Geometry: final body of the model. Coordinates: model frame, mm. A direction names the side the tool comes from. Round coordinates to 2 decimals unless told otherwise and drop trailing zeros. Write each loop counter-clockwise with the first axis right and the second up, starting at its lowest first coordinate (ties: lowest second). Pieces come first, ordered by that corner, then holes.
from build123d import *

# Parameters (mm, degrees)
SKETCH1_R               = 22.5
BOSS_EXTRUDE1_DEPTH     = 50
CUT_EXTRUDE1_REACH      = 130.311
CUT_EXTRUDE1_END_RADIUS = 22.5
SKETCH2_R               = 5


with BuildPart() as part:
    # Sketch1 → Boss-Extrude1 (new body)
    with BuildSketch(Plane.XY):
        with BuildLine():
            Line((45, 56.93759592), (45, 96.93759592))
            Line((45, 96.93759592), (35, 96.93759592))
            Line((35, 96.93759592), (5, 71.764606985))
            Line((5, 71.764606985), (-5, 71.764606985))
            Line((-5, 71.764606985), (-35, 96.93759592))
            Line((-35, 96.93759592), (-45, 96.93759592))
            Line((-45, 96.93759592), (-45, 56.93759592))
            ThreePointArc((-45, 56.93759592), (-26.127859204, 45.841981394), (-28.726666617, 24.104535363))
            ThreePointArc((-28.726666617, 24.104535363), (0, -37.5), (28.726666617, 24.104535363))
            ThreePointArc((28.726666617, 24.104535363), (26.127859204, 45.841981394), (45, 56.93759592))
        make_face()
        Circle(SKETCH1_R, mode=Mode.SUBTRACT)
    extrude(amount=BOSS_EXTRUDE1_DEPTH)

    # Cut-Extrude1: up to this cylinder (the profile starts outside it)
    cut_extrude1_end = Plane(origin=(0, 0, 25), z_dir=(0, 0, -1)) * Cylinder(CUT_EXTRUDE1_END_RADIUS, 306.622, mode=Mode.PRIVATE)
    # Sketch2 → Cut-Extrude1 (cut, up to the surface)
    with BuildSketch(Plane(origin=(0, 71.764606985, 0), x_dir=(1, 0, 0), z_dir=(0, 1, 0)), mode=Mode.PRIVATE) as cut_extrude1_sk1:
        with Locations(Location((0, -25, 0), (0, 0, 180))):
            Circle(SKETCH2_R)
    cut_extrude1_tool1 = extrude(cut_extrude1_sk1.sketch, amount=-CUT_EXTRUDE1_REACH, mode=Mode.PRIVATE) - cut_extrude1_end
    add(cut_extrude1_tool1.solids().sort_by_distance((0, 71.764607, 25))[0], mode=Mode.SUBTRACT)


solid = part.part
1) Draft query along Y for faces 1 (the flat face through (0, 71.765, 10)), 2 (the flat face through (-1, 31, 50)), 3 (the cylindrical face through (-26.274, 46.131, 24.65)). Return one class per face: pulls with the +Y half, pulls with the -Y half, needs draft (parallel to the pull), parting line crosses it, or undercut.
2) Section D-D on z = 12.5. Output: boundary loops of the cut face in (x, y).
3) Reachability of faces 4 (the cylindrical face through (1.08, 47.2, 20.12)), 5 (the flat face through (-19.79, 84.175, 24.65)), 6 (the cylindrical face through (-1.19, -37.48, 24.65)) from +Z, -Z, +X, -X, +Y, -Y: full face, straight path, thin tool, end or side. Return the list, or none.
4) First-contact query: P1, Ø3, axis at x = -1, z = 15.5, coming from the +Y side; P2, Ø1, axis at y = 1.5, z = 19.5, coming from the -X side; P3, Ø8, axis at x = 0, z = 25, coming from the +Y side. Flat tips, straight axial feed; report the tip coordinate or a pass-through.
5) Section C-C on y = 61.5. Output: boundary loops of the cut face in (x, z), plus the area to 3 significant figures.
6) Line query: probe 1 along Z at (x, y) = (0, 61); probe 2 along Y at (x, z) = (1, 15); probe 3 along Y at (x, z) = (6.5, 16). Output: solid intervals per line, ascending.
7) Section B-B on x = 0. Output: boundary loops of the cut face in (y, z), plus the area to 3 significant figures.
8) Section A-A on y = 0. Output: boundary loops of the cut face in (x, z), plus the area to 3 significant figures.
Filled in:
1. face 1: pulls with the +Y half
1. face 2: needs draft
1. face 3: undercut
2. outline: (-45, 56.94) arc R20 cw to (-28.73, 24.1) arc R37.5 ccw (long way) to (28.73, 24.1) arc R20 cw to (45, 56.94) - (45, 96.94) - (35, 96.94) - (5, 71.76) - (-5, 71.76) - (-35, 96.94) - (-45, 96.94) - close; hole circle Ø45 at (0, 0)
3. face 4: +Y
3. face 5: +Z, -Z, +Y
3. face 6: +Z, -Z
4. P1: stops at y = 71.76
4. P2: stops at x = -37.49
4. P3: stops at y = -22.14
5. outline: (-45, 0) - (45, 0) - (45, 50) - (-45, 50) - close; hole circle Ø10 at (0, 25)
5. area: 4,420 mm2
6. probe 1: z = 0 to 20, 30 to 50
6. probe 2: y = -37.49 to -22.48, 22.48 to 71.76
6. probe 3: y = -36.93 to -21.54, 21.54 to 73.02
7. outline: (-37.5, 0) - (-22.5, 0) - (-22.5, 50) - (-37.5, 50) - close; (22.5, 0) - (71.76, 0) - (71.76, 20) - (22.5, 20) - close; (22.5, 30) - (71.76, 30) - (71.76, 50) - (22.5, 50) - close
7. area: 2,720 mm2
8. outline: (-37.5, 0) - (-22.5, 0) - (-22.5, 50) - (-37.5, 50) - close; (22.5, 0) - (37.5, 0) - (37.5, 50) - (22.5, 50) - close
8. area: 1,500 mm2
